CAD build for the part. Positions are in the model's coordinates, mm. Face numbers are marked on the shaded views. A direction names the side the tool comes from. Give positions to 0.01 mm unless a question says otherwise; leave off trailing zeros. Order: outer loops, then holes, each group sorted by start corner. A loop starts at its lowest first (then second) coordinate and runs counter-clockwise, first axis right, second up. Notation, with made-up numbers: (-31.5, -17) -> (-3.5, -17) arc R18 cw to (-3.5, -3) -> close; hole circle Ø6 at (48, 54.5). An arc over 180 degrees is marked (long way). Answer as CSV lines item,"result".
```python
from build123d import *

# Parameters (mm, degrees)
BOSS_EXTRUDE1_DEPTH     = 30
SKETCH3_R               = 2
CUT_EXTRUDE2_DEPTH      = 19.00000001
SKETCH8_R               = 3.5
CUT_EXTRUDE5_DEPTH      = 10
SKETCH9_W               = 8.000001136
SKETCH9_H               = 1
CUT_EXTRUDE6_DEPTH      = 2.999999513
CUT_EXTRUDE6_DEPTH_BACK = 19.00000011
CUT_EXTRUDE7_START      = -3
CUT_EXTRUDE7_DEPTH      = 5.999999514
SKETCH12_R              = 5.08
CUT_EXTRUDE8_DEPTH      = 15


with BuildPart() as part:
    # Sketch1 → Boss-Extrude1 (new body)
    with BuildSketch(Plane.XY):
        with BuildLine():
            Line((7.999999523, 12.236067772), (7.999999523, 7.763931751))
            ThreePointArc((7.999999523, 7.763931751), (10.474207269, 7.037715521), (12.598076062, 8.499999806))
            Line((12.598076062, 8.499999806), (23.999999754, 8.499999806))
            Line((23.999999754, 8.499999806), (23.999999754, 1.999999464))
            Line((23.999999754, 1.999999464), (15.9999988, 1.999999464))
            ThreePointArc((15.9999988, 1.999999464), (-3.4e-08, 9.99999976), (15.999998799, 18.00000006))
            Line((15.999998799, 18.00000006), (23.999999935, 18.00000006))
            Line((23.999999935, 18.00000006), (23.999999935, 11.500000167))
            Line((23.999999935, 11.500000167), (12.598075802, 11.500000167))
            ThreePointArc((12.598075802, 11.500000167), (10.474207012, 12.962284044), (7.999999523, 12.236067772))
        make_face()
    extrude(amount=BOSS_EXTRUDE1_DEPTH)

    # Sketch3 → Cut-Extrude2 (cut, through all)
    with BuildSketch(Plane(origin=(0, 18.00000006, 0), x_dir=(1, 0, 0), z_dir=(0, 1, 0))):
        with Locations((17.999999935, -22.5)):
            Circle(SKETCH3_R)
    cut_extrude2 = extrude(amount=-CUT_EXTRUDE2_DEPTH, mode=Mode.SUBTRACT)

    # Sketch8 → Cut-Extrude5 (cut)
    with BuildSketch(Plane(origin=(0, 18.00000006, 0), x_dir=(1, 0, 0), z_dir=(0, 1, 0))):
        with Locations((17.999999935, -22.5)):
            Circle(SKETCH8_R)
    cut_extrude5 = extrude(amount=CUT_EXTRUDE5_DEPTH, mode=Mode.SUBTRACT)

    # Sketch9 → Cut-Extrude6 (cut, two sides)
    with BuildSketch(Plane(origin=(0, 18.00000006, 0), x_dir=(1, 0, 0), z_dir=(0, 1, 0))) as cut_extrude6_sk:
        with Locations((19.999999367, -15)):
            Rectangle(SKETCH9_W, SKETCH9_H)
    extrude(amount=CUT_EXTRUDE6_DEPTH, mode=Mode.SUBTRACT)
    extrude(cut_extrude6_sk.sketch, amount=-CUT_EXTRUDE6_DEPTH_BACK, mode=Mode.SUBTRACT)

    # Sketch10 → Cut-Extrude7 (cut)
    with BuildSketch(Plane.XZ.offset(-1.999999464).offset(CUT_EXTRUDE7_START)):
        Polygon((15.067996564, 20.882381514), (17.934896952, 19.152001354), (20.866900323, 20.76961984), (20.932003306, 24.117618486), (18.065102919, 25.847998646), (15.133099548, 24.23038016), align=None)
    cut_extrude7 = extrude(amount=CUT_EXTRUDE7_DEPTH, mode=Mode.SUBTRACT)

    # Mirror1: Cut-Extrude7 across plane
    add(cut_extrude7.mirror(Plane.XY.offset(15)), mode=Mode.SUBTRACT)

    # Mirror2: Cut-Extrude2, Cut-Extrude5 across plane
    add(cut_extrude2.mirror(Plane.XY.offset(15)), mode=Mode.SUBTRACT)
    add(cut_extrude5.mirror(Plane.XY.offset(15)), mode=Mode.SUBTRACT)

    # Sketch12 → Cut-Extrude8 (cut)
    with BuildSketch(Plane.XY.offset(30)):
        with Locations((9.999999677, 9.999999762)):
            Circle(SKETCH12_R)
    extrude(amount=-CUT_EXTRUDE8_DEPTH, mode=Mode.SUBTRACT)


solid = part.part
```
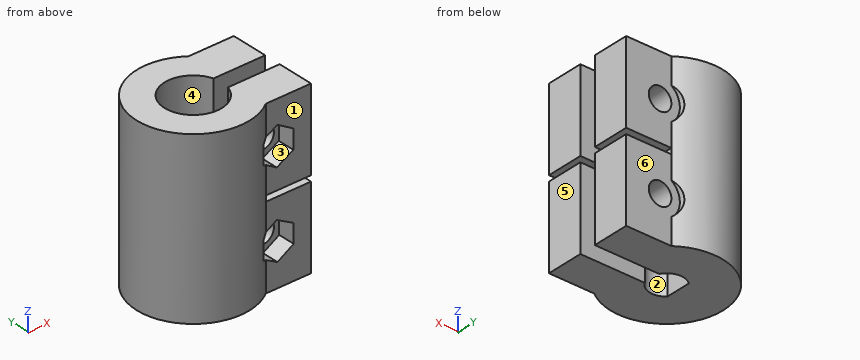
1) Band-saw the part on C-C, the plane y = 16.5. Write the cut outline in (x, z), then the cut area to 3 significant figures.
Data:
outline,"(2.4, 0) -> (24, 0) -> (24, 14.5) -> (16, 14.5) -> (16, 15.5) -> (24, 15.5) -> (24, 30) -> (2.4, 30) -> close; hole circle Ø4 at (18, 7.5); hole circle Ø4 at (18, 22.5)"
area,"615 mm2"
2) Which spindle directions (+Z, -Z, +X, -X, +Y, -Y) get a long thin tool onto all of the face, cutting with end or side? Do the marked faces 1, 2 and 3. Say none if no direction does.
Data:
face 1,"+Z, -Z, +X, -Y"
face 2,"+Z, -Z"
face 3,"-Y"
3) Band-saw the part on B-B, the plane z = 3. Write the cut outline in (x, y), then the cut area to 3 significant figures.
Data:
outline,"(8, 7.76) -> (8, 12.24) arc R3 cw to (12.6, 11.5) -> (24, 11.5) -> (24, 18) -> (16, 18) arc R10 ccw (long way) to (16, 2) -> (24, 2) -> (24, 8.5) -> (12.6, 8.5) arc R3 cw to start"
area,"339 mm2"
4) Wall check: line 1 along Z through (x, y) = (18, 15.75); line 2 along X through (y, z) = (6.9, 22.5); line 3 along Y through (x, z) = (10, 18). Give the ranges that are in metal, low to high. Write a range as [from, to].
Data:
line 1,"z = [0, 5.5], [9.5, 14.5], [15.5, 20.5], [24.5, 30]"
line 2,"x = [0.49, 5.98], [14.02, 16], [20, 24]"
line 3,"y = [0, 4.92], [15.08, 20]"
5) Band-saw the part on D-D, the plane z = 7.5. Write the cut outline in (x, y).
Data:
outline,"(8, 7.76) -> (8, 12.24) arc R3 cw to (12.6, 11.5) -> (16, 11.5) -> (16, 18) -> (14.5, 18) -> (14.5, 18.93) arc R10 ccw (long way) to (15.1, 1.4) -> (15.1, 5) -> (16, 5) -> (16, 8.5) -> (12.6, 8.5) arc R3 cw to start; (20, 5) -> (20.9, 5) -> (20.9, 2) -> (24, 2) -> (24, 8.5) -> (20, 8.5) -> close; (20, 11.5) -> (24, 11.5) -> (24, 18) -> (20, 18) -> close"
6) Band-saw the part on A-A, the plane x = 10. Write the cut outline in (y, z), then the cut area to 3 significant figures.
Data:
outline,"(0, 0) -> (7, 0) -> (7, 15) -> (4.92, 15) -> (4.92, 30) -> (0, 30) -> close; (13, 0) -> (20, 0) -> (20, 30) -> (15.08, 30) -> (15.08, 15) -> (13, 15) -> close"
area,"358 mm2"
7) Pin check, flat tips, straight feed: P1, Ø5, axis at x = 19, z = 25, coming from the +Y side; P2, Ø3.5, axis at x = 16.5, z = 15, coming from the -Y side; P3, Ø12, axis at x = 11, z = 5.5, coming from the -Y side; P4, Ø4.5, axis at x = 17.5, z = 7.5, coming from the -Y side. Stop position of each tip, or through.
Data:
P1,"stops at y = 18"
P2,"stops at y = 1.2"
P3,"stops at y = 0"
P4,"stops at y = 5"
8) Pull direction Y, two halves, no side cores. Call the marked faces 4, 5 and 6: pulls with the +Y half, pulls with the -Y half, needs draft (parallel to the pull), parting line crosses it, or undercut.
Data:
face 4,"undercut"
face 5,"needs draft"
face 6,"pulls with the +Y half"
